Build history of the part. All positions in model axes, mm. Face numbers are marked on the shaded views. Round coordinates to 2 decimals unless told otherwise and drop trailing zeros. Write each loop counter-clockwise with the first axis right and the second up, starting at its lowest first coordinate (ties: lowest second). Pieces come first, ordered by that corner, then holes. Notation, with made-up numbers: (83, 89.25) -> (139, 89.25) arc R18 cw to (139, 99.25) -> close; hole circle Ø1 at (-6.5, 65). An arc over 180 degrees is marked (long way). One line per question, with ' | ' between items.
from build123d import *

# Parameters (mm, degrees)
F0_R     = 25.4
F0_R_2   = 6.35
F1_DEPTH = 25
F2_R     = 5
F3_DEPTH = 50


with BuildPart() as f1:
    # F0 (on Top) → F1 (new body, symmetric)
    with BuildSketch(Plane.XY):
        Circle(F0_R)
        with Locations((-12.990381, -7.5)):
            Circle(F0_R_2, mode=Mode.SUBTRACT)
        with Locations((12.990381, -7.5)):
            Circle(F0_R_2, mode=Mode.SUBTRACT)
        with Locations((0, 15)):
            Circle(F0_R_2, mode=Mode.SUBTRACT)
    extrude(amount=F1_DEPTH, both=True)

    # F2 (on face) → F3 (join)
    with BuildSketch(Plane(origin=(0, 0, -25), x_dir=(1, 0, 0), z_dir=(0, 0, -1))):
        Circle(F2_R)
    extrude(amount=F3_DEPTH)


solid = f1.part
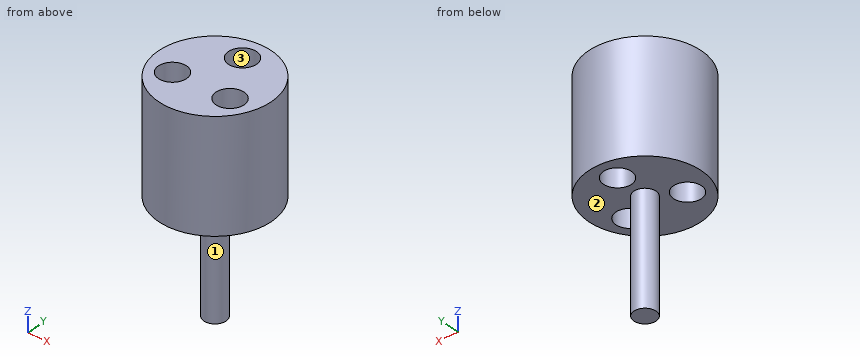
(1) Slice it at B-B (y = 0). Write the cut outline in (x, z).
Calculated:
outline: (-25.4, -25) -> (-5, -25) -> (-5, -75) -> (5, -75) -> (5, -25) -> (25.4, -25) -> (25.4, 25) -> (-25.4, 25) -> close
(2) Mould opens along Y. For the marked faces 1, 2 and 3 say: pulls with the +Y half, pulls with the -Y half, needs draft (parallel to the pull), parting line crosses it, or undercut.
Calculated:
face 1: parting line crosses it | face 2: needs draft | face 3: undercut
(3) Slice it at A-A (x = 8). Write the cut outline in (y, z), then the cut area to 3 significant figures.
Calculated:
outline: (-24.11, -25) -> (-11.43, -25) -> (-11.43, 25) -> (-24.11, 25) -> close; (-3.57, -25) -> (24.11, -25) -> (24.11, 25) -> (-3.57, 25) -> close | area: 2,020 mm2
(4) Slice it at D-D (y = 15). Write the cut outline in (x, z).
Calculated:
outline: (-20.5, -25) -> (-6.35, -25) -> (-6.35, 25) -> (-20.5, 25) -> close; (6.35, -25) -> (20.5, -25) -> (20.5, 25) -> (6.35, 25) -> close
(5) Wall check: line 1 (X direction, y = -7, z = 3); line 2 (Z direction, x = 5.5, y = -16); line 3 (Y direction, x = -9, z = -13). Give the ranges that are in metal, low to high. Write a range as from..to.
Calculated:
line 1: -24.42..-19.32, -6.66..6.66, 19.32..24.42 | line 2: -25..25 | line 3: -23.75..-12.44, -2.56..23.75
(6) Drop flat-ended pins along their axis: pin 1 (8 mm diameter, centred on x = -7.5, y = -4.5, fed in from +Z); pin 2 (1.5 mm diameter, centred on x = 9.5, y = -18.5, fed in from -Z); pin 3 (6 mm diameter, centred on x = 12.5, z = -25, fed in from -Y); pin 4 (5 mm diameter, centred on x = -10.5, z = -13, fed in from -Y). Give the stop position or say it passes through.
Calculated:
pin 1: z = 25 | pin 2: z = -25 | pin 3: y = -23.56 | pin 4: y = -24.11
(7) Slice it at C-C (y = -7.5). Write the cut outline in (x, z).
Calculated:
outline: (-24.27, -25) -> (-19.34, -25) -> (-19.34, 25) -> (-24.27, 25) -> close; (-6.64, -25) -> (6.64, -25) -> (6.64, 25) -> (-6.64, 25) -> close; (19.34, -25) -> (24.27, -25) -> (24.27, 25) -> (19.34, 25) -> close
